Part model, mm, in its own coordinate system. A direction names the side the tool comes from. Give positions to 0.01 mm unless a question says otherwise; leave off trailing zeros. Write each loop counter-clockwise with the first axis right and the second up, starting at its lowest first coordinate (ties: lowest second). Pieces come first, ordered by that corner, then holes.
```python
from build123d import *

# Parameters (mm, degrees)
SKETCH_W        = 62
SKETCH_H        = 52.5
SKETCH_R        = 2.15
SKETCH_W_2      = 40.6
SKETCH_H_2      = 20.2
PAD_DEPTH       = 4
SKETCH001_W     = 62
SKETCH001_H     = 4
PAD001_DEPTH    = 15
PAD002_DEPTH    = 1
FILLET_R        = 4
SKETCH003_R     = 1.6
POCKET_DEPTH    = 4.001
POCKET001_DEPTH = 19.001
FILLET001_R     = 2


with BuildPart() as part:
    # Sketch → Pad (new body)
    with BuildSketch(Plane.XY):
        Rectangle(SKETCH_W, SKETCH_H)
        with Locations((-24.55, 18.5)):
            Circle(SKETCH_R, mode=Mode.SUBTRACT)
        with Locations((-24.55, 8.5)):
            Circle(SKETCH_R, mode=Mode.SUBTRACT)
        with Locations((24.55, 18.5)):
            Circle(SKETCH_R, mode=Mode.SUBTRACT)
        with Locations((24.55, 8.5)):
            Circle(SKETCH_R, mode=Mode.SUBTRACT)
        with Locations((0, 13.75)):
            Rectangle(SKETCH_W_2, SKETCH_H_2, mode=Mode.SUBTRACT)
    extrude(amount=PAD_DEPTH)

    # Sketch001 (on Face13 of Pad) → Pad001 (join)
    with BuildSketch(Plane(origin=(0, 0, 0), x_dir=(1, 0, 0), z_dir=(0, 0, -1))):
        with Locations((0, 24.25)):
            Rectangle(SKETCH001_W, SKETCH001_H)
    extrude(amount=PAD001_DEPTH)

    # Sketch002 (on Face16 of Pad001) → Pad002 (join)
    with BuildSketch(Plane.YZ.offset(31)):
        Polygon((-22.25, 0), (-22.25, -15), (26.25, 0), align=None)
    pad002 = extrude(amount=-PAD002_DEPTH)

    # Mirrored: Pad002 across YZ
    add(pad002.mirror(Plane.YZ))

    # Fillet
    fillet_edges = [part.edges().sort_by_distance(p)[0] for p in [
        (0, -22.25, 0),
    ]]
    fillet(fillet_edges, radius=FILLET_R)

    # Sketch003 (on Face14 of Fillet) → Pocket (cut, through all)
    with BuildSketch(Plane(origin=(0, -22.25, 0), x_dir=(-1, 0, 0), z_dir=(0, 1, 0))):
        with Locations((-20, -9.5)):
            Circle(SKETCH003_R)
        with Locations((20, -9.5)):
            Circle(SKETCH003_R)
        with Locations((0, -9.5)):
            Circle(SKETCH003_R)
    extrude(amount=-POCKET_DEPTH, mode=Mode.SUBTRACT)

    # Sketch005 (on Face19 of Pocket) → Pocket001 (cut, through all)
    with BuildSketch(Plane.XY.offset(4)):
        Polygon((-20.3, 17.25), (-22.1, 17.25), (-23.8, 15.55), (-27.3, 15.55), (-27.3, 11.95), (-23.8, 11.95), (-22.1, 10.25), (-20.3, 10.25), align=None)
        Polygon((20.3, 17.25), (22.1, 17.25), (23.8, 15.55), (27.3, 15.55), (27.3, 11.95), (23.8, 11.95), (22.1, 10.25), (20.3, 10.25), align=None)
    extrude(amount=-POCKET001_DEPTH, mode=Mode.SUBTRACT)

    # Fillet001
    fillet001_edges = [part.edges().sort_by_distance(p)[0] for p in [
        (0, -26.25, 4),
    ]]
    fillet(fillet001_edges, radius=FILLET001_R)


solid = part.part
```
1) Wall check: L1, parallel to X at y = -21.5, z = -11; L2, parallel to Y at x = 24.55, z = 1.9; L3, parallel to Z at x = 0, y = -23.9. Give the ranges that are in metal, low to high.
Answers follow:
L1: x = -31 to -30, 30 to 31
L2: y = -26.25 to 6.35, 10.65 to 11.95, 15.55 to 16.35, 20.65 to 26.25
L3: z = -15 to -11.1, -7.9 to 4
2) Two-plate mould, pull along Y, no slides. Class faces 1 (the face through (0, -4, 4)), 2 (the face through (0, 26.25, 2)), 3 (the face through (20.3, 21, 2)), 4 (the face through (-27.3, 14, 2)): +Y half, -Y half, draft (parallel to the pull), parting line (faces both ways), or undercut.
Answers follow:
face 1: draft
face 2: +Y half
face 3: undercut
face 4: undercut
3) 3-axis set-ups, long thin cutter, end or side, ignore diameter. For faces 5 (the face through (20.35, -24.22, -11.06)), 6 (the face through (-20.3, 7, 2)), 7 (the face through (0, -22.25, -12)): which of +Z, -Z, +X, -X, +Y, -Y reach the whole face in a straight line?
Answers follow:
face 5: +Y, -Y
face 6: +Z, -Z
face 7: -Z, +Y
4) Saw through at B-B, the plane z = 0.75. Write the cut outline in (x, y).
Answers follow:
outline: (-31, -26.25) - (31, -26.25) - (31, 26.25) - (-31, 26.25) - close; hole (-27.3, 11.95) - (-23.8, 11.95) - (-22.1, 10.25) - (-20.3, 10.25) - (-20.3, 3.65) - (20.3, 3.65) - (20.3, 10.25) - (22.1, 10.25) - (23.8, 11.95) - (27.3, 11.95) - (27.3, 15.55) - (23.8, 15.55) - (22.1, 17.25) - (20.3, 17.25) - (20.3, 23.85) - (-20.3, 23.85) - (-20.3, 17.25) - (-22.1, 17.25) - (-23.8, 15.55) - (-27.3, 15.55) - close; hole circle Ø4.3 at (-24.55, 8.5); hole circle Ø4.3 at (-24.55, 18.5); hole circle Ø4.3 at (24.55, 8.5); hole circle Ø4.3 at (24.55, 18.5)
5) Pin check, flat tips, straight feed: pin 1 Ø5.5 at (x, z) = (5.5, -9) entering from +Y; pin 2 Ø8 at (x, y) = (-4, -15.5) entering from -Z; pin 3 Ø4 at (x, y) = (24.55, 8.5) entering from +Z; pin 4 Ø8 at (x, y) = (-15, 7.5) entering from -Z. Stop position of each tip, or through.
Answers follow:
pin 1: stops at y = -22.25
pin 2: stops at z = -0.2
pin 3: passes through
pin 4: stops at z = 0
6) Saw through at D-D, the plane x = 0. Write the cut outline in (y, z), then the cut area to 3 significant figures.
Answers follow:
outline: (-26.25, -15) - (-22.25, -15) - (-22.25, -11.1) - (-26.25, -11.1) - close; (-26.25, -7.9) - (-22.25, -7.9) - (-22.25, -4) arc R4 cw to (-18.25, 0) - (3.65, 0) - (3.65, 4) - (-24.25, 4) arc R2 ccw to (-26.25, 2) - close; (23.85, 0) - (26.25, 0) - (26.25, 4) - (23.85, 4) - close
area: 179 mm2
7) Saw through at A-A, the plane x = -24.55. Write the cut outline in (y, z).
Answers follow:
outline: (-26.25, -15) - (-22.25, -15) - (-22.25, -4) arc R4 cw to (-18.25, 0) - (6.35, 0) - (6.35, 4) - (-24.25, 4) arc R2 ccw to (-26.25, 2) - close; (10.65, 0) - (11.95, 0) - (11.95, 4) - (10.65, 4) - close; (15.55, 0) - (16.35, 0) - (16.35, 4) - (15.55, 4) - close; (20.65, 0) - (26.25, 0) - (26.25, 4) - (20.65, 4) - close
8) Saw through at C-C, the plane y = 18.5. Write the cut outline in (x, z).
Answers follow:
outline: (-31, -2.4) - (-30, -2.4) - (-30, 0) - (-26.7, 0) - (-26.7, 4) - (-31, 4) - close; (-22.4, 0) - (-20.3, 0) - (-20.3, 4) - (-22.4, 4) - close; (20.3, 0) - (22.4, 0) - (22.4, 4) - (20.3, 4) - close; (26.7, 0) - (30, 0) - (30, -2.4) - (31, -2.4) - (31, 4) - (26.7, 4) - close
